Geometry: see drawing. Coordinates: mm, zero at the bounding-box minimum. Give positions to 0.01 mm unless a question says otherwise; leave off trailing zeros. Loops run counter-clockwise (first coordinate to the right, second up) from the corner with the lowest first, then second, coordinate; pieces in that order, holes last. Notation, with made-up numbers: M -14,84.5 L 3,84.5 A7 cw 3,92.5 Z; hole C -6.5,-31.75 d2. An arc over 180 degrees is marked long. Return JSON: item names as keys, results as strings. Group by question number.
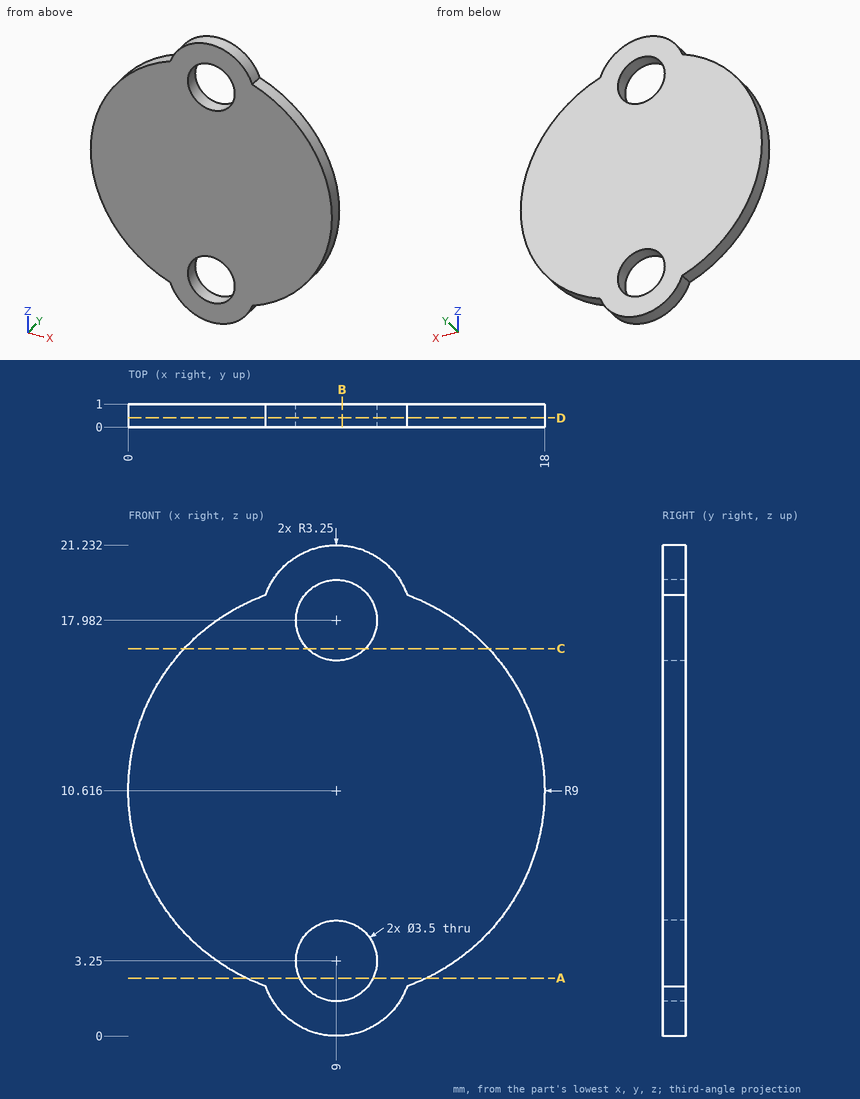
Item 1: Section A-A, the plane z = 2.5. Return loops of the section in (x, y), then the cut area to 3 significant figures.
Item 2: Section B-B, the plane x = 9.25. Return loops of the section in (y, z).
Item 3: Section D-D, the plane y = 0.4. Return loops of the section in (x, z).
Item 4: Section C-C, the plane z = 16.75. Return loops of the section in (x, y), then the cut area to 3 significant figures.
Item 5: First-contact query: pin 1 Ø4 at (x, z) = (8, 4.5) entering from +Y. Flat tip, straight axial feed; report the tip coordinate or a pass-through.
Item 6: Material intervals for line 1 (Z direction, x = 8.75, y = 0.8); line 2 (X direction, y = 0.55, z = 3.75); line 3 (X direction, y = 0.65, z = 4), sorted ascending. Write a range as from..to.
Answer below:
{
 "1": {"outline": "M 5.11,0 L 7.42,0 L 7.42,1 L 5.11,1 Z; M 10.58,0 L 12.89,0 L 12.89,1 L 10.58,1 Z", "area": "4.62 mm^2"},
 "2": {"outline": "M 0,0.01 L 1,0.01 L 1,1.52 L 0,1.52 Z; M 0,4.98 L 1,4.98 L 1,16.25 L 0,16.25 Z; M 0,19.71 L 1,19.71 L 1,21.22 L 0,21.22 Z"},
 "3": {"outline": "M 5.94,2.15 A3.25 ccw 12.06,2.15 A9 ccw 12.06,19.08 A3.25 ccw 5.94,19.08 A9 ccw Z; hole C 9,3.25 d3.5; hole C 9,17.98 d3.5"},
 "4": {"outline": "M 2.41,0 L 7.76,0 L 7.76,1 L 2.41,1 Z; M 10.24,0 L 15.59,0 L 15.59,1 L 10.24,1 Z", "area": "10.7 mm^2"},
 "5": {"pin 1": "y = 1"},
 "6": {"line 1": "0.01..1.52, 4.98..16.25, 19.71..21.22", "line 2": "3.18..7.32, 10.68..14.82", "line 3": "2.9..7.42, 10.58..15.1"}
}
